```python
from build123d import *
from build123d import SkipClean  # not in build123d's __all__

# Parameters (mm, degrees)
F1_DEPTH = 100
F2_R     = 2
F3_DEPTH = 15
F4_R     = 2
F5_DEPTH = 6
F6_DEPTH = 100.0010001
F8_R     = 2
F9_DEPTH = 10


with BuildPart() as f1:
    # F0 (on Top) → F1 (new body)
    with BuildSketch(Plane.XY):
        with BuildLine():
            ThreePointArc((-36.113968879, 21.9828632864), (-38.5839959268, 36.6822584753), (-23.884600738, 34.2122314274))
            Line((-23.884600738, 34.2122314274), (-21.3320395526, 34.2122314274))
            ThreePointArc((-21.3320395526, 34.2122314274), (-40.2456968626, 38.3439594111), (-36.113968879, 19.430302101))
            Line((-36.113968879, 19.430302101), (-36.113968879, 21.9828632864))
        make_face()
        with BuildLine():
            ThreePointArc((-23.884600738, 34.2122314274), (-23.1970967118, 32.2645205774), (-22.963968879, 30.2122314274))
            ThreePointArc((-22.963968879, 30.2122314274), (-27.2599756775, 22.4558630762), (-36.113968879, 21.9828632864))
            Line((-36.113968879, 21.9828632864), (-36.113968879, 19.430302101))
            ThreePointArc((-36.113968879, 19.430302101), (-25.5470061107, 20.7716276332), (-20.613968879, 30.2122314274))
            ThreePointArc((-20.613968879, 30.2122314274), (-20.7949100123, 32.2442024836), (-21.3320395526, 34.2122314274))
            Line((-21.3320395526, 34.2122314274), (-23.884600738, 34.2122314274))
        make_face()
        with BuildLine():
            ThreePointArc((-52.113968879, 30.2122314274), (-46.2561045027, 44.3543670512), (-32.113968879, 50.2122314274))
            Line((-32.113968879, 50.2122314274), (-52.113968879, 50.2122314274))
            Line((-52.113968879, 50.2122314274), (-52.113968879, 30.2122314274))
        make_face()
        with BuildLine():
            ThreePointArc((-32.113968879, 50.2122314274), (-19.4648582383, 45.7041648123), (-12.5180509367, 34.2122314274))
            ThreePointArc((-12.5180509367, 34.2122314274), (-12.2152458189, 32.2224106675), (-12.113968879, 30.2122314274))
            Line((-12.113968879, 30.2122314274), (-12.113968879, 50.2122314274))
            Line((-12.113968879, 50.2122314274), (-32.113968879, 50.2122314274))
        make_face()
        with BuildLine():
            Line((-12.113968879, 10.2122314274), (-12.113968879, 30.2122314274))
            ThreePointArc((-12.113968879, 30.2122314274), (-17.9718332553, 16.0700958037), (-32.113968879, 10.2122314274))
            Line((-32.113968879, 10.2122314274), (-12.113968879, 10.2122314274))
        make_face()
        with BuildLine():
            ThreePointArc((-32.113968879, 10.2122314274), (-34.1241481191, 10.3135083673), (-36.113968879, 10.6163134852))
            ThreePointArc((-36.113968879, 10.6163134852), (-47.6059022638, 17.5631207868), (-52.113968879, 30.2122314274))
            Line((-52.113968879, 30.2122314274), (-52.113968879, 10.2122314274))
            Line((-52.113968879, 10.2122314274), (-32.113968879, 10.2122314274))
        make_face()
        with BuildLine():
            ThreePointArc((-36.113968879, 15.7553991326), (-42.7205705968, 40.8188331452), (-17.6571365842, 34.2122314274))
            Line((-17.6571365842, 34.2122314274), (-12.5180509367, 34.2122314274))
            ThreePointArc((-12.5180509367, 34.2122314274), (-19.4648582383, 45.7041648123), (-32.113968879, 50.2122314274))
            ThreePointArc((-32.113968879, 50.2122314274), (-46.2561045027, 44.3543670512), (-52.113968879, 30.2122314274))
            ThreePointArc((-52.113968879, 30.2122314274), (-47.6059022638, 17.5631207868), (-36.113968879, 10.6163134852))
            Line((-36.113968879, 10.6163134852), (-36.113968879, 15.7553991326))
        make_face()
        with BuildLine():
            Line((-12.5180509367, 34.2122314274), (-17.6571365842, 34.2122314274))
            ThreePointArc((-17.6571365842, 34.2122314274), (-17.2503810816, 32.2305866462), (-17.113968879, 30.2122314274))
            ThreePointArc((-17.113968879, 30.2122314274), (-23.0310178167, 18.2748950411), (-36.113968879, 15.7553991326))
            Line((-36.113968879, 15.7553991326), (-36.113968879, 10.6163134852))
            ThreePointArc((-36.113968879, 10.6163134852), (-34.1241481191, 10.3135083673), (-32.113968879, 10.2122314274))
            ThreePointArc((-32.113968879, 10.2122314274), (-17.9718332553, 16.0700958037), (-12.113968879, 30.2122314274))
            ThreePointArc((-12.113968879, 30.2122314274), (-12.2152458189, 32.2224106675), (-12.5180509367, 34.2122314274))
        make_face()
        with BuildLine():
            ThreePointArc((-36.113968879, 19.430302101), (-40.2456968626, 38.3439594111), (-21.3320395526, 34.2122314274))
            Line((-21.3320395526, 34.2122314274), (-17.6571365842, 34.2122314274))
            ThreePointArc((-17.6571365842, 34.2122314274), (-42.7205705968, 40.8188331452), (-36.113968879, 15.7553991326))
            Line((-36.113968879, 15.7553991326), (-36.113968879, 19.430302101))
        make_face()
    extrude(amount=F1_DEPTH)

    # F2 (on face) → F3 (cut)
    with BuildSketch(Plane.XZ.offset(-10.2122314274)):
        with Locations((-32.113968879, 85)):
            Circle(F2_R)
    extrude(amount=-F3_DEPTH, mode=Mode.SUBTRACT)

    # F4 (on face) → F5 (cut)
    with BuildSketch(Plane.YZ.offset(-12.113968879)):
        with Locations((30.2122314274, 15)):
            Circle(F4_R)
    extrude(amount=-F5_DEPTH, mode=Mode.SUBTRACT)

    # F0 (on Top) → F6 (cut, through all)
    with BuildSketch(Plane.XY):
        with BuildLine():
            Line((-12.113968879, 10.2122314274), (-12.113968879, 30.2122314274))
            ThreePointArc((-12.113968879, 30.2122314274), (-17.9718332553, 16.0700958037), (-32.113968879, 10.2122314274))
            Line((-32.113968879, 10.2122314274), (-12.113968879, 10.2122314274))
        make_face()
        with BuildLine():
            ThreePointArc((-32.113968879, 10.2122314274), (-34.1241481191, 10.3135083673), (-36.113968879, 10.6163134852))
            ThreePointArc((-36.113968879, 10.6163134852), (-47.6059022638, 17.5631207868), (-52.113968879, 30.2122314274))
            Line((-52.113968879, 30.2122314274), (-52.113968879, 10.2122314274))
            Line((-52.113968879, 10.2122314274), (-32.113968879, 10.2122314274))
        make_face()
        with BuildLine():
            ThreePointArc((-52.113968879, 30.2122314274), (-46.2561045027, 44.3543670512), (-32.113968879, 50.2122314274))
            Line((-32.113968879, 50.2122314274), (-52.113968879, 50.2122314274))
            Line((-52.113968879, 50.2122314274), (-52.113968879, 30.2122314274))
        make_face()
        with BuildLine():
            ThreePointArc((-32.113968879, 50.2122314274), (-19.4648582383, 45.7041648123), (-12.5180509367, 34.2122314274))
            ThreePointArc((-12.5180509367, 34.2122314274), (-12.2152458189, 32.2224106675), (-12.113968879, 30.2122314274))
            Line((-12.113968879, 30.2122314274), (-12.113968879, 50.2122314274))
            Line((-12.113968879, 50.2122314274), (-32.113968879, 50.2122314274))
        make_face()
    with SkipClean():  # cleaning this boolean's faces spoils the solid; the shape is the same uncleaned
        extrude(amount=F6_DEPTH, mode=Mode.SUBTRACT)

    # F8 (on offset) → F9 (cut)
    with BuildSketch(Plane.YZ.offset(-30)):
        with Locations((30.0163067877, 85.1406082511)):
            Circle(F8_R)
    with SkipClean():  # cleaning this boolean's faces spoils the solid; the shape is the same uncleaned
        extrude(amount=F9_DEPTH, mode=Mode.SUBTRACT)


solid = f1.part
```
The model under review builds one solid part; all positions refer to its coordinate system, in mm. A direction names the side the tool comes from. Round coordinates to 2 decimals unless told otherwise and drop trailing zeros. Order: outer loops, then holes, each group sorted by start corner. A loop starts at its lowest first (then second) coordinate and runs counter-clockwise, first axis right, second up. Notation, with made-up numbers: (-34.75, 63.25) -> (-3.75, 63.25) arc R29 ccw to (-3.75, 98.25) -> close; hole circle Ø11 at (22.25, -13). An arc over 180 degrees is marked (long way). Use a Markdown table: item, result.
Q1. We need section B-B on x = -28.5. Write out the cut boundary in (y, z).
Values:
| item | result |
|---|---|
| outline | (10.54, 0) -> (15.65, 0) -> (15.65, 100) -> (10.54, 100) -> close; (19.29, 0) -> (21.81, 0) -> (21.81, 100) -> (19.29, 100) -> close; (38.62, 0) -> (49.88, 0) -> (49.88, 100) -> (38.62, 100) -> close |
Q2. We need section A-A on z = 60.5. Write out the cut boundary in (x, y).
Values:
| item | result |
|---|---|
| outline | circle Ø40 at (-32.11, 30.21); hole circle Ø18.3 at (-32.11, 30.21); hole (-36.11, 15.76) arc R15 ccw to (-17.66, 34.21) -> (-21.33, 34.21) arc R11.5 cw to (-36.11, 19.43) -> close |
Q3. Mouldability with a two-part tool opening along Z and no side actions: class faces 5 (the flat face through (-41, 35, 100)), 6 (the flat face through (-41, 35, 0)), 7 (the cylindrical face through (-32.374, 12.745, 86.983)) as +Z half, -Z half, draft (parallel to the pull), parting line (faces both ways), or undercut.
Values:
| item | result |
|---|---|
| face 5 | +Z half |
| face 6 | -Z half |
| face 7 | undercut |
Q4. We need section D-D on y = 45.5. Write out the cut boundary in (x, z), then the cut area to 3 significant figures.
Values:
| item | result |
|---|---|
| outline | (-45.01, 0) -> (-19.22, 0) -> (-19.22, 100) -> (-45.01, 100) -> close |
| area | 2,580 mm^2 |
Q5. We need section C-C on z = 15. Write out the cut boundary in (x, y).
Values:
| item | result |
|---|---|
| outline | (-36.11, 15.76) -> (-36.11, 19.43) arc R11.5 ccw to (-21.33, 34.21) -> (-17.66, 34.21) arc R15 cw to (-17.25, 32.21) -> (-12.21, 32.21) arc R20 ccw (long way) to (-12.21, 28.21) -> (-17.25, 28.21) arc R15 cw to start; hole circle Ø18.3 at (-32.11, 30.21) |
Q6. For line 1 (X direction, y = 30, z = 54.5); line 2 (X direction, y = 30, z = 84.5); line 3 (X direction, y = 29, z = 54.5), list the stretches that pass through material, from the lowest coordinate up.
Values:
| item | result |
|---|---|
| line 1 | x = -52.11 to -41.26, -22.97 to -20.62, -17.12 to -12.12 |
| line 2 | x = -52.11 to -41.26, -17.12 to -12.12 |
| line 3 | x = -52.08 to -41.18, -23.04 to -20.68, -17.16 to -12.15 |
Q7. Clearance check with flat-ended pins moving along their axes: P1, Ø2, axis at x = -18, z = 55.5, coming from the +Y side; P2, Ø3, axis at y = 17.5, z = 48.5, coming from the +X side; P3, Ø10, axis at x = -42.5, z = 39, coming from the +Y side. State where each tip first meets the part, or that it passes through.
Values:
| item | result |
|---|---|
| P1 | stops at y = 45.31 |
| P2 | stops at x = -15.55 |
| P3 | stops at y = 49.47 |
Q8. Tool access review of faces 1 (the cylindrical face through (-21.94, 31.86, 84.37)), 2 (the flat face through (-36.114, 18, 49)), 3 (the cylindrical face through (-14.645, 28.738, 16.352)), 4 (the cylindrical face through (-34.11, 19.98, 85.09)): name each direction out of +Z, -Z, +X, -X, +Y, -Y from which nothing blocks a thin tool from reaching the whole face with its end or side.
Values:
| item | result |
|---|---|
| face 1 | none |
| face 2 | +Z, -Z |
| face 3 | +X |
| face 4 | -Y |
